from build123d import *

# Parameters (mm, degrees)
SKETCH2_OUTSIDE_W   = 57.892
SKETCH2_OUTSIDE_H   = 57.892
SKETCH2_OUTSIDE_W_2 = 30
SKETCH2_OUTSIDE_H_2 = 42
CUT_EXTRUDE1_DEPTH  = 10
DIAMETERHOLE1_D     = 4.5
TAP1_REACH          = 56.286
TAP1_BORE_R         = 2.4585


with BuildPart() as part:
    # Sketch1 → Revolve1 (revolve)
    with BuildSketch(Plane.XY, mode=Mode.PRIVATE) as revolve1_sk:
        with BuildLine():
            Line((-28, 8), (-28, 11))
            ThreePointArc((-28, 11), (-27.707106781, 11.707106781), (-27, 12))
            Line((-27, 12), (0, 12))
            Line((0, 12), (0, 20.5))
            ThreePointArc((0, 20.5), (0.146446609, 20.853553391), (0.5, 21))
            Line((0.5, 21), (7.5, 21))
            ThreePointArc((7.5, 21), (7.853553391, 20.853553391), (8, 20.5))
            Line((8, 20.5), (8, 8))
            Line((8, 8), (7.5, 8))
            Line((7.5, 8), (7.5, 7.75))
            Line((7.5, 7.75), (8, 7.75))
            Line((8, 7.75), (8, 6))
            Line((8, 6), (-28, 6))
            Line((-28, 6), (-28, 7.75))
            Line((-28, 7.75), (-27.5, 7.75))
            Line((-27.5, 7.75), (-27.5, 8))
            Line((-27.5, 8), (-28, 8))
        make_face()
    revolve(revolve1_sk.sketch.rotate(Axis((-29.8, 0, 0), (1, 0, 0)), 90), axis=Axis((-29.8, 0, 0), (1, 0, 0)))

    # Sketch2 outside → Cut-Extrude1 (cut)
    with BuildSketch(Plane(origin=(8, 0, 0), x_dir=(0, 0, -1), z_dir=(1, 0, 0))):
        Rectangle(SKETCH2_OUTSIDE_W, SKETCH2_OUTSIDE_H)
        Rectangle(SKETCH2_OUTSIDE_W_2, SKETCH2_OUTSIDE_H_2, mode=Mode.SUBTRACT)
    extrude(amount=-CUT_EXTRUDE1_DEPTH, mode=Mode.SUBTRACT)

    # DiameterHole1 (through all)
    with Locations(Plane(origin=(8, 0, 0), x_dir=(0, 0, -1), z_dir=(1, 0, 0))):
        with Locations((11.313708499, 11.313708499), (0, 16), (-11.313708499, 11.313708499), (-11.313708499, -11.313708499), (0, -16), (11.313708499, -11.313708499)):
            Hole(DIAMETERHOLE1_D / 2)

    # Tap1 bore → Tap1 (cut, up to next)
    with BuildSketch(Plane(origin=(0, 19.401470183, 8.03635208), x_dir=(1, 0, 0), z_dir=(0, 0.9238795325112865, 0.3826834323650906)), mode=Mode.PRIVATE) as tap1_sk1:
        with Locations((4, 0)):
            Circle(TAP1_BORE_R)
    tap1_tool1 = extrude(tap1_sk1.sketch, amount=-TAP1_REACH, mode=Mode.PRIVATE) & part.part
    add(tap1_tool1.solids().sort_by_distance((4, 19.40147, 8.036352))[0], mode=Mode.SUBTRACT)


solid = part.part
Geometry: final body of the model. Coordinates: model frame, mm. A direction names the side the tool comes from. Round coordinates to 2 decimals unless told otherwise and drop trailing zeros. Loops run counter-clockwise (first coordinate to the right, second up) from the corner with the lowest first, then second, coordinate; pieces in that order, holes last.
Q1. Access query for faces 1 (the cylindrical face through (7.753, -7.684, -1.009)), 2 (the flat face through (0, 9, -10)), 3 (the cylindrical face through (6.27, 11.97, 5.98)). Directions: +Z, -Z, +X, -X, +Y, -Y. A direction counts if a zero-diameter tool reaches every point of the face in a straight line with its end or side. Return the directions, or none.
Q2. Pin query (flat end, axial travel): P1, Ø8, axis at x = -22.5, z = 1.5, coming from the +Y side; P2, Ø5, axis at y = 16, z = 0, coming from the -X side; P3, Ø5, axis at y = 1.5, z = -3, coming from the +X side; P4, Ø6, axis at x = -11, z = 8, coming from the +Y side. Return the tip coordinate at first contact, or that it passes through.
Q3. Material intervals for L1, parallel to Y at x = -27.8, z = 0; L2, parallel to Y at x = -27.55, z = 0; L3, parallel to Y at x = -13, z = 5.5, sorted ascending.
Q4. Pull-direction query (Z, two-part tool) for faces 4 (the cylindrical face through (-13.311, -3.604, 11.446)), 5 (the cylindrical face through (3.94, -13.31, 12.35)), 6 (the flat face through (8, 5, 4)); classes: released by +Z, released by -Z, zero draft, split by the parting line, or undercut.
Q5. Section B-B on x = -8. Return loops of the section in (y, z), plus the area to 3 significant figures.
Q6. Section C-C on y = 16. State how many separate pieces and enclosed holes the cut face has, plus the area to 3 significant figures.
Evaluation:
1. face 1: +X
1. face 2: -X
1. face 3: none
2. P1: stops at y = 12
2. P2: stops at x = 0
2. P3: passes through
2. P4: stops at y = 10.91
3. L1: y = -11.6 to -8, -7.75 to -6, 6 to 7.75, 8 to 11.6
3. L2: y = -11.84 to -8, -7.75 to -6, 6 to 7.75, 8 to 11.84
3. L3: y = -10.67 to -2.4, 2.4 to 10.67
4. face 4: split by the parting line
4. face 5: undercut
4. face 6: zero draft
5. outline: circle Ø24 at (0, 0); hole circle Ø12 at (0, 0)
5. area: 339 mm2
6. separate pieces: 2
6. enclosed holes: 1
6. area: 161 mm2
